Part print with two shaded views. Sizes in mm from the minimum x, y, z corner. A direction names the side the tool comes from. Coordinates: 2 decimals unless noted, no trailing zeros. Write each loop counter-clockwise with the first axis right and the second up, starting at its lowest first coordinate (ties: lowest second). Pieces come first, ordered by that corner, then holes. Notation, with made-up numbers: (63.25, 82.25) - (109.25, 82.25) arc R11 ccw to (109.25, 89.25) - close; hole circle Ø8 at (67, 47). An arc over 180 degrees is marked (long way). One line per question, with ' | ' between items. Start each with the question number.
1. Probe line 1 (X direction, y = 17.5, z = 3.25); line 2 (X direction, y = 21, z = 2.5); line 3 (X direction, y = 24.75, z = 14.5). List the from-to ranges inside material, lowest first.
2. Flat gauge pins, fed straight in: P1, Ø7.5, axis at x = 9.652, y = 18.796, coming from the +Z side; P2, Ø2, axis at y = 21, z = 19.5, coming from the -X side; P3, Ø10, axis at x = 36, y = 17, coming from the +Z side. Where does each tip first touch, or does it go through?
3. Band-saw the part on C-C, the plane y = 4.5. Write the cut outline in (x, z), then the cut area to 3 significant figures.
4. Two-plate mould, pull along X, no slides. Class the marked faces 1, 2, 3 and 4: +X half, -X half, draft (parallel to the pull), parting line (faces both ways), or undercut.
5. Band-saw the part on D-D, the plane y = 19.75. Write the cut outline in (x, z), then the cut area to 3 significant figures.
6. Band-saw the part on A-A, the plane z = 13.5. Write the cut outline in (x, y).
7. Band-saw the part on B-B, the plane x = 9. Write the cut outline in (y, z).
8. Which spindle directions (+Z, -Z, +X, -X, +Y, -Y) get a long thin tool onto all of the face, cutting with end or side? Do the marked faces 5, 6 and 7. Say none if no direction does.
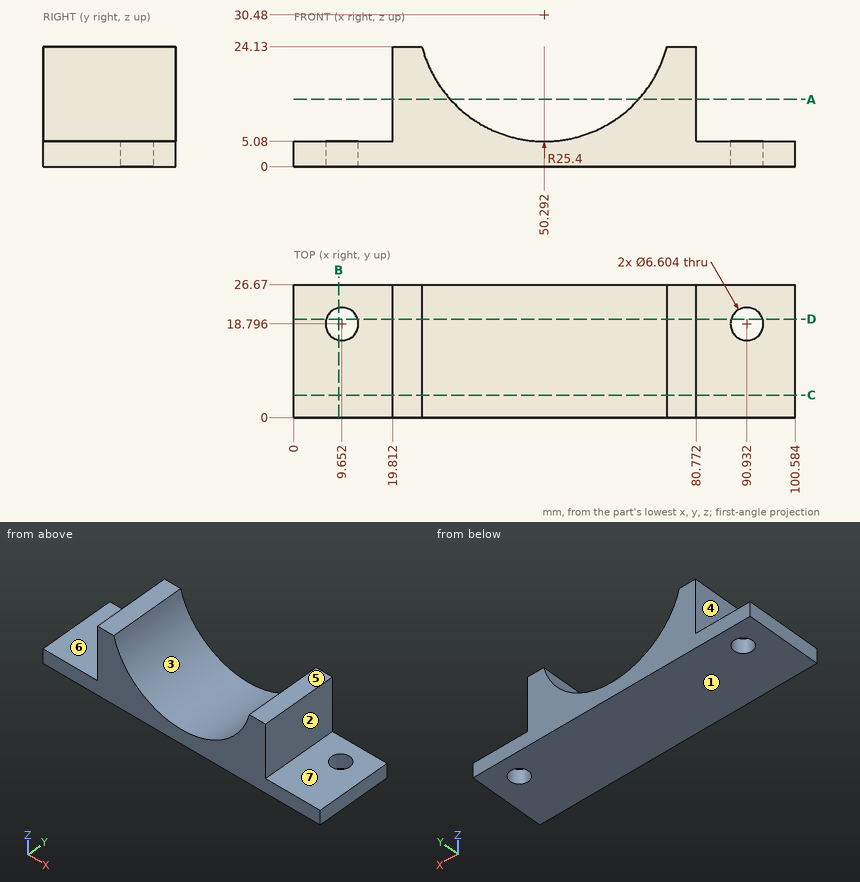
Filled in:
1) line 1: x = 0 to 6.61, 12.69 to 87.89, 93.97 to 100.58 | line 2: x = 0 to 7.19, 12.11 to 88.47, 93.39 to 100.58 | line 3: x = 19.81 to 30.55, 70.04 to 80.77
2) P1: stops at z = 5.08 | P2: stops at x = 19.81 | P3: stops at z = 13.96
3) outline: (0, 0) - (100.58, 0) - (100.58, 5.08) - (80.77, 5.08) - (80.77, 24.13) - (74.89, 24.13) arc R25.4 cw to (25.7, 24.13) - (19.81, 24.13) - (19.81, 5.08) - (0, 5.08) - close | area: 978 mm²
4) face 1: draft | face 2: +X half | face 3: undercut | face 4: -X half
5) outline: (0, 0) - (6.49, 0) - (6.49, 5.08) - (0, 5.08) - close; (12.81, 0) - (87.77, 0) - (87.77, 5.08) - (80.77, 5.08) - (80.77, 24.13) - (74.89, 24.13) arc R25.4 cw to (25.7, 24.13) - (19.81, 24.13) - (19.81, 5.08) - (12.81, 5.08) - close; (94.09, 0) - (100.58, 0) - (100.58, 5.08) - (94.09, 5.08) - close | area: 914 mm²
6) outline: (19.81, 0) - (31.4, 0) - (31.4, 26.67) - (19.81, 26.67) - close; (69.18, 0) - (80.77, 0) - (80.77, 26.67) - (69.18, 26.67) - close
7) outline: (0, 0) - (15.56, 0) - (15.56, 5.08) - (0, 5.08) - close; (22.03, 0) - (26.67, 0) - (26.67, 5.08) - (22.03, 5.08) - close
8) face 5: +Z, +X, -X, +Y, -Y | face 6: +Z, -X, +Y, -Y | face 7: +Z, +X, +Y, -Y
